Model file for the job. Use its own axes, mm. Round coordinates to 2 decimals unless told otherwise and drop trailing zeros. Loops run counter-clockwise (first coordinate to the right, second up) from the corner with the lowest first, then second, coordinate; pieces in that order, holes last. Notation, with made-up numbers: M 5.5,-7 L 48.5,-7 A16 cw 48.5,24 Z; hole C -13,15 d5. An arc over 180 degrees is marked long. Answer in a Markdown table with one row per item.
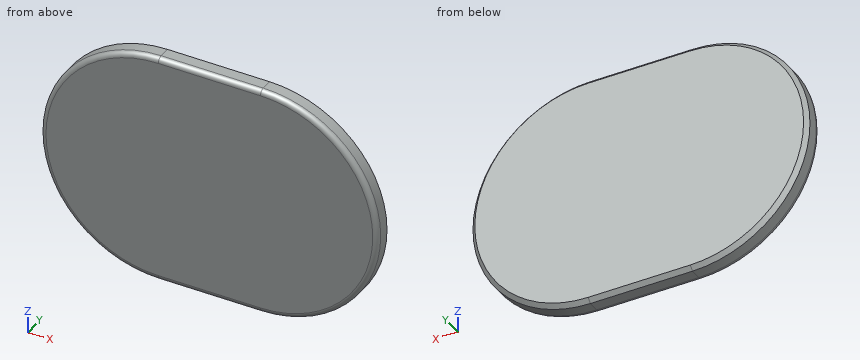
from build123d import *

# Parameters (mm, degrees)
BOSS_EXTRUDE1_DEPTH = 4
CHAMFER1_SIZE       = 0.8
FILLET1_R           = 1


with BuildPart() as part:
    # Sketch1 → Boss-Extrude1 (new body)
    with BuildSketch(Plane(origin=(0, 0, 0), x_dir=(1, 0, 0), z_dir=(0, 1, 0))):
        with BuildLine():
            Line((-10, 23), (10, 23))
            ThreePointArc((10, 23), (33, 0), (10, -23))
            Line((10, -23), (-10, -23))
            ThreePointArc((-10, -23), (-33, 0), (-10, 23))
        make_face()
    extrude(amount=BOSS_EXTRUDE1_DEPTH)

    # Chamfer1
    chamfer1_edges = [part.edges().sort_by_distance(p)[0] for p in [
        (33, 4, 0),
        (0, 4, -23),
        (-33, 4, 0),
        (0, 4, 23),
    ]]
    chamfer(chamfer1_edges, length=CHAMFER1_SIZE)

    # Fillet1
    fillet1_edges = [part.edges().sort_by_distance(p)[0] for p in [
        (0, 0, -23),
        (33, 0, 0),
        (0, 0, 23),
        (-33, 0, 0),
    ]]
    fillet(fillet1_edges, radius=FILLET1_R)


solid = part.part
1. Pin check, flat tip, straight feed: pin 1 (1 mm diameter, centred on y = 3, z = 6.5, fed in from +X). Stop position of the tip, or through.
Verdict:
| item | result |
|---|---|
| pin 1 | stops at x = 32.2 |
2. Wall check: probe 1 along X at (y, z) = (1.95, -5.5); probe 2 along X at (y, z) = (1.1, 9); probe 3 along Z at (x, y) = (18, 1.5). Give the ranges that are in metal, low to high.
Verdict:
| item | result |
|---|---|
| probe 1 | x = -32.33 to 32.33 |
| probe 2 | x = -31.17 to 31.17 |
| probe 3 | z = -21.56 to 21.56 |
3. Saw through at A-A (y = 2.1). Write the cut outline in (x, z), and give its area (3 significant figures).
Verdict:
| item | result |
|---|---|
| outline | M -10,-23 L 10,-23 A23 ccw 10,23 L -10,23 A23 ccw Z |
| area | 2,580 mm² |
